Verification items for the finished model (mm, model axes). A direction names the side the tool comes from. Give positions to 0.01 mm unless a question says otherwise; leave off trailing zeros. Loops run counter-clockwise (first coordinate to the right, second up) from the corner with the lowest first, then second, coordinate; pieces in that order, holes last. Notation, with made-up numbers: (12, 50) -> (18, 50) arc R19 cw to (18, 63) -> close; hole circle Ø7 at (-30.5, 46.25). An arc over 180 degrees is marked (long way). Use one line per item in the form item = value. Start each with the question number.
from build123d import *

# Parameters (mm, degrees)
BOSS_EXTRU_1_DEPTH           = 4
ESQUISSE3_R                  = 7.26
BOSS_EXTRU_2_DEPTH           = 1.9
ENL_V_MAT_EXTRU_1_DEPTH      = 29.119468345
ENL_V_MAT_EXTRU_1_DEPTH_BACK = 29.119468345
ESQUISSE2_R                  = 1.65
BOSS_EXTRU_3_START           = 1.85
ESQUISSE4_R                  = 1.65
BOSS_EXTRU_3_DEPTH           = 1.85
CONG_1_R                     = 10
ESQUISSE5_R                  = 3
ENL_V_MAT_EXTRU_2_DEPTH      = 2.84


with BuildPart() as part:
    # Esquisse1 → Boss.-Extru.1 (new body)
    with BuildSketch(Plane(origin=(0, 0, 0), x_dir=(1, 0, 0), z_dir=(0, 1, 0))):
        with BuildLine():
            Line((-3.245, 6.494426457), (-3.245, 23.625))
            ThreePointArc((-3.245, 23.625), (0, 26.87), (3.245, 23.625))
            Line((3.245, 23.625), (3.245, 6.494426457))
            ThreePointArc((3.245, 6.494426457), (0, -7.26), (-3.245, 6.494426457))
        make_face()
    extrude(amount=BOSS_EXTRU_1_DEPTH)

    # Esquisse3 → Boss.-Extru.2 (add)
    with BuildSketch(Plane(origin=(0, 4, 0), x_dir=(1, 0, 0), z_dir=(0, 1, 0))):
        with Locations(Location((0, 0, 0), (0, 0, 63.450571564))):
            Circle(ESQUISSE3_R)
    extrude(amount=BOSS_EXTRU_2_DEPTH)

    # Esquisse2 → Enlèv. mat.-Extru.1 (cut, two sides: drawn at the far end of the back side and taken through both)
    with BuildSketch(Plane(origin=(0, 4, 0), x_dir=(1, 0, 0), z_dir=(0, 1, 0)).offset(-ENL_V_MAT_EXTRU_1_DEPTH_BACK)):
        with Locations(Location((0, 0, 0), (0, 0, 270))):
            Circle(ESQUISSE2_R)
        with Locations(Location((0, 19.28, 0), (0, 0, 270))):
            Circle(ESQUISSE2_R)
        with Locations(Location((0, 24.02, 0), (0, 0, 270))):
            Circle(ESQUISSE2_R)
    extrude(amount=ENL_V_MAT_EXTRU_1_DEPTH + ENL_V_MAT_EXTRU_1_DEPTH_BACK, mode=Mode.SUBTRACT)

    # Esquisse4 → Boss.-Extru.3 (add)
    with BuildSketch(Plane(origin=(0, 4, 0), x_dir=(1, 0, 0), z_dir=(0, 1, 0)).offset(BOSS_EXTRU_3_START)):
        with BuildLine():
            ThreePointArc((1.394847662, 21.65), (0, 26.77), (-1.394847662, 21.65))
            ThreePointArc((-1.394847662, 21.65), (0, 16.53), (1.394847662, 21.65))
        make_face()
        with Locations(Location((0, 24.02, 0), (0, 0, 270))):
            Circle(ESQUISSE4_R, mode=Mode.SUBTRACT)
        with Locations(Location((0, 19.28, 0), (0, 0, 270))):
            Circle(ESQUISSE4_R, mode=Mode.SUBTRACT)
    extrude(amount=-BOSS_EXTRU_3_DEPTH)

    # Congé1
    # the kernel refuses this fillet: 10 mm, written as the material it adds along each edge
    with BuildSketch(Plane(origin=(3.245, 0, -6.494426457), x_dir=(0, 0, -1), z_dir=(0, 1, 0))) as cong_1_piece_1:
        with BuildLine():
            CenterArc((4.572532249, -10), CONG_1_R, 90, 39.880695656)
            ThreePointArc((-1.839378936, -2.326187717), (-0.799649919, -1.258012346), (0, 0))
            Line((0, 0), (4.572532249, 0))
        make_face()
    extrude(amount=4)
    with BuildSketch(Plane(origin=(-3.245, 0, -6.494426457), x_dir=(0, 0, -1), z_dir=(0, 1, 0))) as cong_1_piece_2:
        with BuildLine():
            CenterArc((4.572532249, 10), CONG_1_R, 230.119304344, 39.880695656)
            ThreePointArc((-1.839378936, 2.326187717), (-0.799649919, 1.258012346), (0, 0))
            Line((0, 0), (4.572532249, 0))
        make_face()
    extrude(amount=4)

    # Esquisse5 → Enlèv. mat.-Extru.2 (cut)
    with BuildSketch(Plane(origin=(0, 5.9, 0), x_dir=(1, 0, 0), z_dir=(0, 1, 0))):
        with Locations(Location((0, 0, 0), (0, 0, 270))):
            Circle(ESQUISSE5_R)
    extrude(amount=-ENL_V_MAT_EXTRU_2_DEPTH, mode=Mode.SUBTRACT)


solid = part.part
Item 1: Sectioned sample at C-C, the plane y = 0.7. Enter the section's corners in (x, z) (3 decimals), and give its area (3 significant figures).
Item 2: Material ranges on line 1 (Z direction, x = 0, y = 1.05); line 2 (X direction, y = 3.9, z = 0); line 3 (X direction, y = 4.8, z = -24.02), recorded low to high.
Item 3: Tool access check on faces 1 (the flat face through (0, 4, -13)), 2 (the flat face through (3.245, 2, -17)), 3 (the flat face through (-3.245, 2, -17)). Record the directions out of +Z, -Z, +X, -X, +Y, -Y that give a thin tool (end or side, any length) a straight path to the whole face; none if there is none.
Item 4: Draft check along X on faces 4 (the flat face through (-1.3, 3.06, 1.3)), 5 (the cylindrical face through (-0.07, 1.97, -26.87)), 6 (the cylindrical face through (3.83, 1.97, -7.7)), 7 (the flat face through (0, 5.85, -22)). Enter one of: +X half, -X half, draft (parallel to the pull), parting line (faces both ways), or undercut.
Item 5: Sectioned sample at D-D, the plane z = 0. Enter the section's corners in (x, y).
Item 6: Sectioned sample at B-B, the plane x = 0. Enter the section's corners in (y, z).
Item 7: Gauge pin test, flat ends, axial feed: pin 1 Ø4 at (x, z) = (0, -19.28) entering from +Y; pin 2 Ø1.2 at (y, z) = (2.5, -17) entering from +X (3 decimals); pin 3 Ø1.2 at (y, z) = (2, -16.5) entering from -X (3 decimals). Record the tip position at first contact, or that the pin passes through.
Item 8: Sectioned sample at A-A, the plane z = -19.28. Enter the section's corners in (x, y) (3 decimals).
Outcome:
q1.outline = (-5.571, -4.655) arc R10 cw to (-3.245, -11.067) -> (-3.245, -23.625) arc R3.245 ccw to (3.245, -23.625) -> (3.245, -11.067) arc R10 cw to (5.571, -4.655) arc R7.26 ccw (long way) to start; hole circle Ø3.3 at (0, -24.02); hole circle Ø3.3 at (0, -19.28); hole circle Ø3.3 at (0, 0)
q1.area = 269 mm^2
q2.line_1 = -26.87 to -25.67, -22.37 to -20.93, -17.63 to -1.65, 1.65 to 7.26
q2.line_2 = -7.26 to -3, 3 to 7.26
q2.line_3 = -2.75 to -1.65, 1.65 to 2.75
q3.face_1 = +Y
q3.face_2 = -Z, +X, +Y, -Y
q3.face_3 = -Z, -X, +Y, -Y
q4.face_4 = undercut
q4.face_5 = parting line
q4.face_6 = +X half
q4.face_7 = draft
q5.outline = (-7.26, 0) -> (-1.65, 0) -> (-1.65, 3.06) -> (-3, 3.06) -> (-3, 5.9) -> (-7.26, 5.9) -> close; (1.65, 0) -> (7.26, 0) -> (7.26, 5.9) -> (3, 5.9) -> (3, 3.06) -> (1.65, 3.06) -> close
q6.outline = (0, -26.87) -> (4, -26.87) -> (4, -26.77) -> (5.85, -26.77) -> (5.85, -25.67) -> (0, -25.67) -> close; (0, -22.37) -> (5.85, -22.37) -> (5.85, -20.93) -> (0, -20.93) -> close; (0, -17.63) -> (5.85, -17.63) -> (5.85, -16.53) -> (4, -16.53) -> (4, -7.26) -> (5.9, -7.26) -> (5.9, -3) -> (3.06, -3) -> (3.06, -1.65) -> (0, -1.65) -> close; (0, 1.65) -> (3.06, 1.65) -> (3.06, 3) -> (5.9, 3) -> (5.9, 7.26) -> (0, 7.26) -> close
q7.pin_1 = 5.85
q7.pin_2 = 3.245
q7.pin_3 = -3.245
q8.outline = (-3.245, 0) -> (-1.65, 0) -> (-1.65, 5.85) -> (-2.75, 5.85) -> (-2.75, 4) -> (-3.245, 4) -> close; (1.65, 0) -> (3.245, 0) -> (3.245, 4) -> (2.75, 4) -> (2.75, 5.85) -> (1.65, 5.85) -> close
